Source: CAD feature listing. Evaluate the final solid. Frame: model axes, mm. Round coordinates to 2 decimals unless told otherwise and drop trailing zeros. Write each loop counter-clockwise with the first axis right and the second up, starting at its lowest first coordinate (ties: lowest second). Pieces come first, ordered by that corner, then holes. Notation, with made-up numbers: (-19, -16.5) -> (-1, -16.5) arc R25 cw to (-1, 18.5) -> close; hole circle Ø2 at (72.25, -26). An arc over 180 degrees is marked (long way). Return JSON: item names as keys, results as strings. Group by question number.
from build123d import *

# Parameters (mm, degrees)
BOSS_EXTRUDE1_DEPTH = 15
SKETCH7_R           = 140
CUT_EXTRUDE3_DEPTH  = 15


with BuildPart() as part:
    # Sketch1 → Boss-Extrude1 (new body)
    with BuildSketch(Plane.XY):
        with BuildLine():
            Line((-112.416665105, 111.821845345), (249.583334895, 111.821845345))
            ThreePointArc((249.583334895, 111.821845345), (280.696033267, 98.934543717), (293.583334895, 67.821845345))
            Line((293.583334895, 67.821845345), (293.583334895, -394.178154655))
            ThreePointArc((293.583334895, -394.178154655), (280.696033267, -425.290853027), (249.583334895, -438.178154655))
            Line((249.583334895, -438.178154655), (-112.416665105, -438.178154655))
            ThreePointArc((-112.416665105, -438.178154655), (-143.529363477, -425.290853027), (-156.416665105, -394.178154655))
            Line((-156.416665105, -394.178154655), (-156.416665105, 67.821845345))
            ThreePointArc((-156.416665105, 67.821845345), (-143.529363477, 98.934543717), (-112.416665105, 111.821845345))
        make_face()
    extrude(amount=BOSS_EXTRUDE1_DEPTH)

    # Sketch7 → Cut-Extrude3 (cut)
    with BuildSketch(Plane.XY.offset(15)):
        with Locations((12.913034287, -269.02154253)):
            Circle(SKETCH7_R)
    extrude(amount=-CUT_EXTRUDE3_DEPTH, mode=Mode.SUBTRACT)


solid = part.part
Item 1: Cut plane C-C on z = 2.5. Output: boundary loops of the cut face in (x, y).
Item 2: Material intervals for probe 1 along X at (y, z) = (-272.5, 13); probe 2 along Y at (x, z) = (-110, 11.5); probe 3 along X at (y, z) = (-188, 11.25), sorted ascending.
Item 3: Cut plane B-B on x = 18. Output: boundary loops of the cut face in (y, z).
Item 4: Pull-direction query (X, two-part tool) for faces 1 (the flat face through (-156.417, -166, 7)), 2 (the flat face through (72, -98, 0)), 3 (the flat face through (293.583, -160, 7)), 4 (the cylindrical face through (-17.4, -405.7, 7.6)); classes: +X half, -X half, draft (parallel to the pull), parting line (faces both ways), or undercut.
Item 5: Cut plane A-A on y = -158.5. Output: boundary loops of the cut face in (x, z).
Here are the results:
{
 "1": {"outline": "(-156.42, -394.18) arc R44 ccw to (-112.42, -438.18) -> (249.58, -438.18) arc R44 ccw to (293.58, -394.18) -> (293.58, 67.82) arc R44 ccw to (249.58, 111.82) -> (-112.42, 111.82) arc R44 ccw to (-156.42, 67.82) -> close; hole circle Ø280 at (12.91, -269.02)"},
 "2": {"probe 1": "x = -156.42 to -127.04, 152.87 to 293.58", "probe 2": "y = -438.18 to -336.05, -202 to 111.82", "probe 3": "x = -156.42 to -101.26, 127.09 to 293.58"},
 "3": {"outline": "(-438.18, 0) -> (-408.93, 0) -> (-408.93, 15) -> (-438.18, 15) -> close; (-129.11, 0) -> (111.82, 0) -> (111.82, 15) -> (-129.11, 15) -> close"},
 "4": {"face 1": "-X half", "face 2": "draft", "face 3": "+X half", "face 4": "undercut"},
 "5": {"outline": "(-156.42, 0) -> (-73.02, 0) -> (-73.02, 15) -> (-156.42, 15) -> close; (98.85, 0) -> (293.58, 0) -> (293.58, 15) -> (98.85, 15) -> close"}
}
